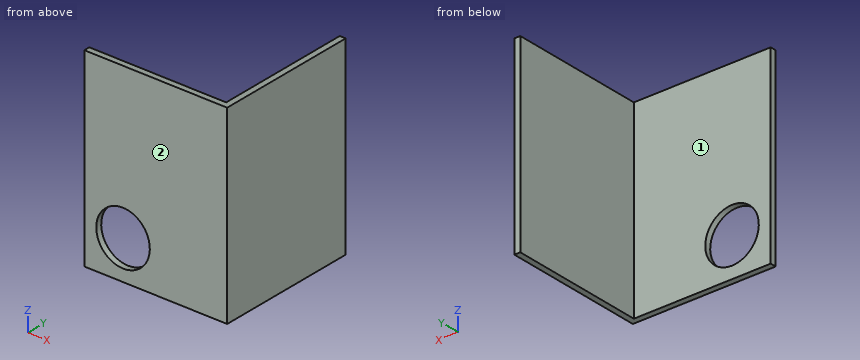
Autodesk Inventor part; units mm, degrees
ref_plane "YZ Plane" through (0, 0, 0) normal (1, 0, 0) x (0, 1, 0)
ref_plane "XZ Plane" through (0, 0, 0) normal (0, 1, 0) x (-1, 0, 0)
ref_plane "XY Plane" through (0, 0, 0) normal (0, 0, 1) x (1, 0, 0)
sketch "Sketch1" plane through (0, 0, 0) normal (0, 0, 1) x (1, 0, 0)
  line L0 (0, 0) -> (76.2, 0)
  line L1 (76.2, 0) -> (76.2, 76.2)
  line L2 (76.2, 76.2) -> (0, 76.2)
  line L3 (0, 3.175) -> (0, 0)
  line L4 (3.175, 3.175) -> (73.025, 3.175)
  line L5 (73.025, 3.175) -> (73.025, 73.025)
  line L6 (3.175, 3.175) -> (0, 3.175)
  line L7 (73.025, 73.025) -> (73.025, 76.2)
  dimension "d0" = 76.2
  dimension "d1" = 76.2
extrude "Extrusion1" add sketch "Sketch1" along normal blind 101.6
sketch "Sketch2" plane through (0, 0, 0) normal (0, -1, 0) x (1, 0, 0)
  line L0 (0, 101.6) -> (76.2, 101.6)
  line L1 (0, 0) -> (0, 101.6)
  point P0 (20.6375, 20.6375)
  dimension "d5" = 80.9625
  dimension "d6" = 20.6375
  dimension "d14" = 101.6
hole "Hole1" at (20.6375, 0, 20.6375) direction (0, 1, 0) diameter 28.575 depth 25.4 tip angle 118
properties part number "ARM_068_NewLongShaftMountFlipped" material "Aluminum 6061"
Check sheet for the modelled part. Datum: model origin and axes. Units: mm. Face numbers are marked on the shaded views. A direction names the side the tool comes from. Give positions to 0.01 mm unless a question says otherwise; leave off trailing zeros. Loops run counter-clockwise (first coordinate to the right, second up) from the corner with the lowest first, then second, coordinate; pieces in that order, holes last. Notation, with made-up numbers: M -4.75,59 L 34.25,59 A18 ccw 34.25,92 Z; hole C 16,41 d2. An arc over 180 degrees is marked long. Answer as CSV lines item,"result".
Item 1: Sectioned sample at C-C, the plane z = 57. Enter the section's corners in (x, y) (3 decimals).
Reply:
outline,"M 0,0 L 76.2,0 L 76.2,76.2 L 73.025,76.2 L 73.025,3.175 L 0,3.175 Z"
Item 2: Depth check by flat-ended pin: pin 1 Ø4 at (y, z) = (11.5, 46) entering from -X (3 decimals); pin 2 Ø22 at (x, z) = (28, 32.5) entering from +Y (3 decimals). Enter the tip coordinate at first touch or a pass-through.
Reply:
pin 1,"x = 73.025"
pin 2,"y = 3.175"
Item 3: Sectioned sample at A-A, the plane x = 26. Enter the section's corners in (y, z) (3 decimals).
Reply:
outline,"M 0,0 L 3.175,0 L 3.175,7.395 L 0,7.395 Z; M 0,33.88 L 3.175,33.88 L 3.175,101.6 L 0,101.6 Z"
Item 4: Set-up check for the marked faces 1 and 2: record each of +Z, -Z, +X, -X, +Y, -Y from which the full face is reachable in a straight line by a thin tool's end or side.
Reply:
face 1,"+Z, -Z, -X, +Y"
face 2,"+Z, -Z, +X, -X, -Y"
Item 5: Sectioned sample at D-D, the plane y = 22. Enter the section's corners in (x, z) (3 decimals).
Reply:
outline,"M 73.025,0 L 76.2,0 L 76.2,101.6 L 73.025,101.6 Z"
Item 6: Scan lines: L1, parallel to Y at x = 5, z = 36 (3 decimals); L2, parallel to X at y = 49, z = 62 (3 decimals). Record each from-to range of solid material in increasing order.
Reply:
L1,"0 to 3.175"
L2,"73.025 to 76.2"
Item 7: Sectioned sample at B-B, the plane z = 16. Enter the section's corners in (x, y) (3 decimals).
Reply:
outline,"M 0,0 L 7.124,0 L 7.124,3.175 L 0,3.175 Z; M 34.151,0 L 76.2,0 L 76.2,76.2 L 73.025,76.2 L 73.025,3.175 L 34.151,3.175 Z"
